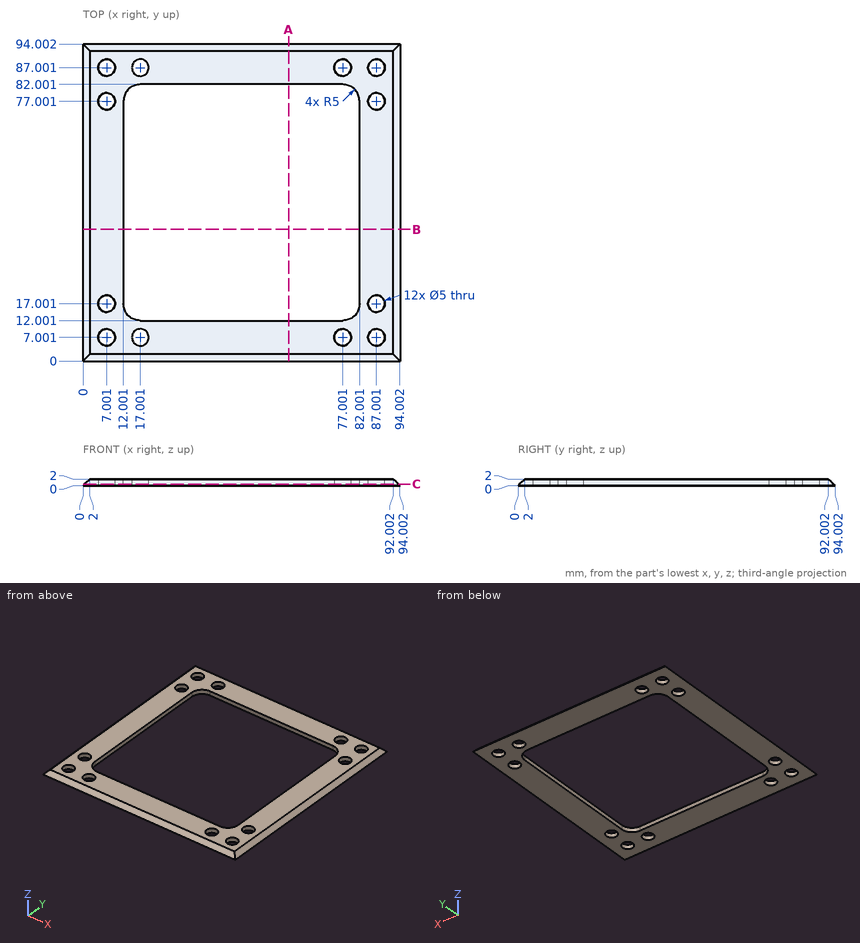
The drawing under review shows one solid part. Ordinate dimensions are in mm from its lowest x, y, z. Round coordinates to 2 decimals unless told otherwise and drop trailing zeros. Loops run counter-clockwise (first coordinate to the right, second up) from the corner with the lowest first, then second, coordinate; pieces in that order, holes last. Notation, with made-up numbers: M 32.5,-15 L 80.5,-15 A31 ccw 80.5,23 Z; hole C 66,40.5 d3. An arc over 180 degrees is marked long. Answer as CSV lines item,"result". Start each with the question number.
Item 1: Wall thickness on line 1 (Y direction, x = 87, z = 0.3); line 2 (Y direction, x = 77, z = 1.4); line 3 (X direction, y = 18, z = 1.35): over which ranges is each line inside the solid? List them lowest first. Write a range as [from, to].
Item 2: Consider section C-C (z = 0.5). State how many separate pieces and enclosed holes the cut face has, then the cut area to 3 significant figures.
Item 3: Insertion check: P1, Ø4.5, axis at x = 17.001, y = 7.001, coming from the +Z side; P2, Ø1, axis at x = 53, z = 1.5, coming from the -Y side. Each pin has a flat end and moves straight along its axis. Give the tip position at first contact, or say it passes through.
Item 4: Consider section A-A (x = 61). Write out the cut boundary in (y, z), then the cut area to 3 significant figures.
Answer:
1,line 1,"y = [0.3, 4.5], [9.5, 14.5], [19.5, 74.5], [79.5, 84.5], [89.5, 93.7]"
1,line 2,"y = [1.4, 4.5], [9.5, 12], [82, 84.5], [89.5, 92.6]"
1,line 3,"x = [1.35, 4.71], [9.29, 12], [82, 84.71], [89.29, 92.65]"
2,separate pieces,"1"
2,enclosed holes,"13"
2,area,"3,540 mm^2"
3,P1,"passes through"
3,P2,"stops at y = 1"
4,outline,"M 0,0 L 12,0 L 12,2 L 2,2 Z; M 82,0 L 94,0 L 92,2 L 82,2 Z"
4,area,"44.0 mm^2"
